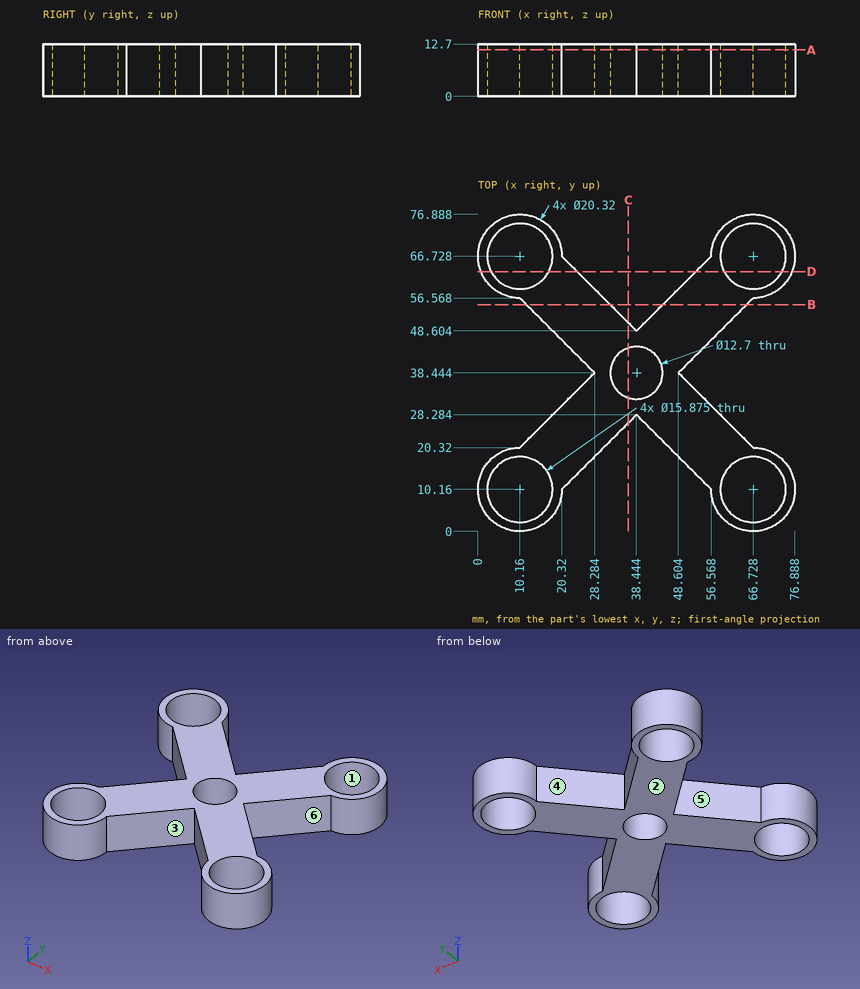
Geometry check sheet. Reference: drawing and pictorial views, mm from the part's lowest x, y, z. A direction names the side the tool comes from. Round coordinates to 2 decimals unless told otherwise and drop trailing zeros. Order: outer loops, then holes, each group sorted by start corner. A loop starts at its lowest first (then second) coordinate and runs counter-clockwise, first axis right, second up. Notation, with made-up numbers: (-3.5, 64.25) - (1.5, 64.25) arc R18 ccw to (1.5, 97.25) - close; hole circle Ø8 at (56.25, -40). An arc over 180 degrees is marked (long way). Write item = value, one per line.
Q1. Section check D-D (y = 63). Record the boundary of the cut face in (x, z) (1 decimal), and give its area (3 significant figures).
Computed:
outline = (0.7, 0) - (3.2, 0) - (3.2, 12.7) - (0.7, 12.7) - close; (17.2, 0) - (24, 0) - (24, 12.7) - (17.2, 12.7) - close; (52.8, 0) - (59.7, 0) - (59.7, 12.7) - (52.8, 12.7) - close; (73.7, 0) - (76.2, 0) - (76.2, 12.7) - (73.7, 12.7) - close
area = 237 mm^2
Q2. Go/stop test with flat-tipped pins: pin 1 (3 mm diameter, centred on x = 46, z = 6, fed in from -Y); pin 2 (2 mm diameter, centred on x = 64.5, z = 2.5, fed in from -Y) (1 decimal); pin 3 (3 mm diameter, centred on x = 27.5, z = 3, fed in from +Y). Record where each tip stops, or that it passes through.
Computed:
pin_1 = 19.23
pin_2 = 0.1
pin_3 = 61.05
Q3. Section check C-C (x = 36.5). Record the boundary of the cut face in (y, z).
Computed:
outline = (26.34, 0) - (32.4, 0) - (32.4, 12.7) - (26.34, 12.7) - close; (44.49, 0) - (50.55, 0) - (50.55, 12.7) - (44.49, 12.7) - close
Q4. Section check A-A (z = 11.25). State how many separate pieces and enclosed holes the cut face has, and give its area (3 significant figures).
Computed:
separate_pieces = 1
enclosed_holes = 5
area = 1,940 mm^2
Q5. Draft check along Y on the marked faces 1, 2 and 3. Enter one of: pulls with the +Y half, pulls with the -Y half, needs draft (parallel to the pull), parting line crosses it, or undercut.
Computed:
face_1 = undercut
face_2 = needs draft
face_3 = pulls with the -Y half
Q6. Tool access check on the marked faces 4, 5 and 6. Record the directions out of +Z, -Z, +X, -X, +Y, -Y that give a thin tool (end or side, any length) a straight path to the whole face; none if there is none.
Computed:
face_4 = +Z, -Z, +Y
face_5 = +Z, -Z, -X
face_6 = +Z, -Z, +X
Q7. Section check B-B (y = 55). Record the boundary of the cut face in (x, z).
Computed:
outline = (11.73, 0) - (32.05, 0) - (32.05, 12.7) - (11.73, 12.7) - close; (44.84, 0) - (65.16, 0) - (65.16, 12.7) - (44.84, 12.7) - close
Q8. Thickness scan on line 1 along X through (y, z) = (67, 4.25) (1 decimal); line 2 along X through (y, z) = (69, 5.25) (1 decimal); line 3 along Y through (x, z) = (23.5, 8.25). Record the ranges inside material, lowest first.
Computed:
line_1 = 0 to 2.2, 18.1 to 20.3, 56.6 to 58.8, 74.7 to 76.9
line_2 = 0.3 to 2.6, 17.8 to 20.1, 56.8 to 59.1, 74.3 to 76.6
line_3 = 13.34 to 33.66, 43.23 to 63.55
